from build123d import *

# Parameters (mm, degrees)
ESQUISSE1_R             = 145
ESQUISSE1_R_2           = 2
ESQUISSE1_W             = 6
ESQUISSE1_H             = 6
BOSS_EXTRU_1_DEPTH      = 6
ESQUISSE2_W             = 17.5
ESQUISSE2_H             = 55
ESQUISSE2_W_2           = 3
ESQUISSE2_H_2           = 8
ESQUISSE2_W_3           = 8
ESQUISSE2_H_3           = 3
ENL_V_MAT_EXTRU_1_DEPTH = 6
CONG_1_R                = 5


with BuildPart() as part:
    # Esquisse1 → Boss.-Extru.1 (new body)
    with BuildSketch(Plane.XY):
        Circle(ESQUISSE1_R)
        with Locations((-37.5, 0)):
            Circle(ESQUISSE1_R_2, mode=Mode.SUBTRACT)
        with Locations((-20, -33)):
            Circle(ESQUISSE1_R_2, mode=Mode.SUBTRACT)
        with Locations((20, -33)):
            Circle(ESQUISSE1_R_2, mode=Mode.SUBTRACT)
        with Locations((20, 33)):
            Circle(ESQUISSE1_R_2, mode=Mode.SUBTRACT)
        with Locations((-20, 33)):
            Circle(ESQUISSE1_R_2, mode=Mode.SUBTRACT)
        with Locations((37.5, 0)):
            Circle(ESQUISSE1_R_2, mode=Mode.SUBTRACT)
        with Locations((0, -46.909918854)):
            Rectangle(ESQUISSE1_W, ESQUISSE1_H, mode=Mode.SUBTRACT)
        with Locations((0, 46.909918854)):
            Rectangle(ESQUISSE1_W, ESQUISSE1_H, mode=Mode.SUBTRACT)
        with Locations((-44.5, 0)):
            Rectangle(ESQUISSE1_W, ESQUISSE1_H, mode=Mode.SUBTRACT)
        with Locations((-30.5, 0)):
            Rectangle(ESQUISSE1_W, ESQUISSE1_H, mode=Mode.SUBTRACT)
        with Locations((-27, -33)):
            Rectangle(ESQUISSE1_W, ESQUISSE1_H, mode=Mode.SUBTRACT)
        with Locations((-13, -33)):
            Rectangle(ESQUISSE1_W, ESQUISSE1_H, mode=Mode.SUBTRACT)
        with Locations((13, -33)):
            Rectangle(ESQUISSE1_W, ESQUISSE1_H, mode=Mode.SUBTRACT)
        with Locations((27, -33)):
            Rectangle(ESQUISSE1_W, ESQUISSE1_H, mode=Mode.SUBTRACT)
        with Locations((13, 33)):
            Rectangle(ESQUISSE1_W, ESQUISSE1_H, mode=Mode.SUBTRACT)
        with Locations((27, 33)):
            Rectangle(ESQUISSE1_W, ESQUISSE1_H, mode=Mode.SUBTRACT)
        with Locations((-27, 33)):
            Rectangle(ESQUISSE1_W, ESQUISSE1_H, mode=Mode.SUBTRACT)
        with Locations((-13, 33)):
            Rectangle(ESQUISSE1_W, ESQUISSE1_H, mode=Mode.SUBTRACT)
        with Locations((30.5, 0)):
            Rectangle(ESQUISSE1_W, ESQUISSE1_H, mode=Mode.SUBTRACT)
        with Locations((44.5, 0)):
            Rectangle(ESQUISSE1_W, ESQUISSE1_H, mode=Mode.SUBTRACT)
    extrude(amount=BOSS_EXTRU_1_DEPTH)

    # Esquisse2 → Enlèv. mat.-Extru.1 (cut)
    with BuildSketch(Plane.XY.offset(6)):
        with Locations((-18.75, 0)):
            Rectangle(ESQUISSE2_W, ESQUISSE2_H)
        with Locations((18.75, 0)):
            Rectangle(ESQUISSE2_W, ESQUISSE2_H)
        with Locations((76, 36)):
            Rectangle(ESQUISSE2_W_2, ESQUISSE2_H_2)
        with Locations((94, 36)):
            Rectangle(ESQUISSE2_W_2, ESQUISSE2_H_2)
        with Locations((76, -36)):
            Rectangle(ESQUISSE2_W_2, ESQUISSE2_H_2)
        with Locations((94, -36)):
            Rectangle(ESQUISSE2_W_2, ESQUISSE2_H_2)
        with Locations((-85, -47.5)):
            Rectangle(ESQUISSE2_W_3, ESQUISSE2_H_3)
        with Locations((-85, 65.5)):
            Rectangle(ESQUISSE2_W_3, ESQUISSE2_H_3)
        with Locations((-85, 47.5)):
            Rectangle(ESQUISSE2_W_3, ESQUISSE2_H_3)
        with Locations((-85, -65.5)):
            Rectangle(ESQUISSE2_W_3, ESQUISSE2_H_3)
        with BuildLine():
            Line((-32.555083478, 55.362694963), (-32.555083478, 115.362694963))
            ThreePointArc((-32.555083478, 115.362694963), (-20.055083478, 127.862694963), (-7.555083478, 115.362694963))
            Line((-7.555083478, 115.362694963), (-7.555083478, 55.362694963))
            ThreePointArc((-7.555083478, 55.362694963), (-20.055083478, 42.862694963), (-32.555083478, 55.362694963))
        make_face()
    extrude(amount=-ENL_V_MAT_EXTRU_1_DEPTH, mode=Mode.SUBTRACT)

    # Congé1
    cong_1_edges = [part.edges().sort_by_distance(p)[0] for p in [
        (27.5, 27.5, 3),
        (10, 27.5, 3),
        (27.5, -27.5, 3),
        (10, -27.5, 3),
        (-27.5, -27.5, 3),
        (-27.5, 27.5, 3),
        (-10, 27.5, 3),
        (-10, -27.5, 3),
    ]]
    fillet(cong_1_edges, radius=CONG_1_R)


solid = part.part
CAD build for the part. Positions are in the model's coordinates, mm. A direction names the side the tool comes from. Give positions to 0.01 mm unless a question says otherwise; leave off trailing zeros. Order: outer loops, then holes, each group sorted by start corner. A loop starts at its lowest first (then second) coordinate and runs counter-clockwise, first axis right, second up. Notation, with made-up numbers: (-2, 61) - (17, 61) arc R24 ccw to (17, 97) - close; hole circle Ø7 at (85.25, -6). An arc over 180 degrees is marked (long way). Answer in a Markdown table with one row per item.
1. Saw through at D-D, the plane x = -94. Give the cut face in (y, z).
Data:
| item | result |
|---|---|
| outline | (-110.4, 0) - (110.4, 0) - (110.4, 6) - (-110.4, 6) - close |
2. Saw through at A-A, the plane y = -15.5. Give the cut face in (x, z).
Data:
| item | result |
|---|---|
| outline | (-144.17, 0) - (-27.5, 0) - (-27.5, 6) - (-144.17, 6) - close; (-10, 0) - (10, 0) - (10, 6) - (-10, 6) - close; (27.5, 0) - (144.17, 0) - (144.17, 6) - (27.5, 6) - close |
3. Saw through at B-B, the plane y = 88. Give the cut face in (x, z), plus the area to 3 significant figures.
Data:
| item | result |
|---|---|
| outline | (-115.24, 0) - (-32.56, 0) - (-32.56, 6) - (-115.24, 6) - close; (-7.56, 0) - (115.24, 0) - (115.24, 6) - (-7.56, 6) - close |
| area | 1,230 mm² |
4. Tool access for faces 4 (the flat face through (-2, 2, 0)), 5 (the cylindrical face through (-20.33, 127.86, 3.04)): list every direction of +Z, -Z, +X, -X, +Y, -Y with a clear straight run to the whole face (end or side of a thin tool).
Data:
| item | result |
|---|---|
| face 4 | -Z, +X, -X, +Y, -Y |
| face 5 | +Z, -Z |
5. Flat gauge pins, fed straight in: pin 1 (1.8 mm diameter, centred on x = -84.5, z = 2.5, fed in from +Y); pin 2 (1 mm diameter, centred on y = 42.5, z = 2, fed in from +X); pin 3 (1.5 mm diameter, centred on x = -34.5, z = 4.5, fed in from +Y). Where does each tip first touch, or does it go through?
Data:
| item | result |
|---|---|
| pin 1 | stops at y = 118.47 |
| pin 2 | stops at x = 138.78 |
| pin 3 | stops at y = 141.02 |
6. Saw through at C-C, the plane z = 1.2. Count the separate pieces of the cut face and the enclosed holes in it, plus the area to 3 significant figures.
Data:
| item | result |
|---|---|
| separate pieces | 1 |
| enclosed holes | 29 |
| area | 61,400 mm² |
7. Pull direction X, two halves, no side cores. Call faces 1 (the cylindrical face through (-19.78, 42.866, 3.042)), 2 (the cylindrical face through (138.304, 43.554, 2.958)), 3 (the flat face through (-2, 2, 6)): pulls with the +X half, pulls with the -X half, needs draft (parallel to the pull), parting line crosses it, or undercut.
Data:
| item | result |
|---|---|
| face 1 | undercut |
| face 2 | parting line crosses it |
| face 3 | needs draft |
8. Probe probe 1 along X at (y, z) = (36.5, 1.35); probe 2 along Y at (x, z) = (-20, 3.1); probe 3 along X at (y, z) = (11.5, 4.7). List the from-to ranges inside material, lowest first. Write a range as [from, to].
Data:
| item | result |
|---|---|
| probe 1 | x = [-140.33, 74.5], [77.5, 92.5], [95.5, 140.33] |
| probe 2 | y = [-143.61, -35], [-31, -27.5], [27.5, 31], [35, 42.86], [127.86, 143.61] |
| probe 3 | x = [-144.54, -27.5], [-10, 10], [27.5, 144.54] |
